Work out the finished part from the listing and answer in its coordinate system (mm). A direction names the side the tool comes from. Round coordinates to 2 decimals unless told otherwise and drop trailing zeros. Order: outer loops, then holes, each group sorted by start corner. A loop starts at its lowest first (then second) coordinate and runs counter-clockwise, first axis right, second up. Notation, with made-up numbers: (75.5, -13.5) - (80.5, -13.5) arc R35 ccw to (80.5, 25.5) - close; hole circle Ø6 at (31.25, 85). An arc over 180 degrees is marked (long way). Use one line per item in the form item = value. Start each with the question number.
Q1. Find the intervals of material crossed by line 1 (Z direction, x = 100, y = 1.55); line 2 (Z direction, x = 6, y = 2.05); line 3 (X direction, y = 0.8, z = -65), in increasing order. Write a range as [from, to].
Q2. Which of the six approach directions +Z, -Z, +X, -X, +Y, -Y give full straight-line access (tool end or side, diameter ignored) to faces 1 (the cylindrical face through (-92.85, 1.48, -71.89)), 2 (the flat face through (-134.558, 1.479, 0.347))?
Q3. For a pull along X with two mould halves and no side action, classify faces 3 (the flat face through (-2, 3, -3)), 4 (the flat face through (134.17, 1.48, 0.91)), 5 (the cylindrical face through (87.15, 1.48, -47.91)) as +X half, -X half, draft (parallel to the pull), parting line (faces both ways), or undercut.
Q4. The part is cut by section A-A on x = 0. Determine the outline of the cut face in (y, z), plus the area to 4 significant figures.
Q5. Given P1, Ø1.5, axis at x = -8, y = 1.5, coming from the -Z side; P2, Ø1.5, axis at y = 1.5, z = -21.5, coming from the -X side; P3, Ø0.9, axis at x = -126.5, y = 1.5, coming from the -Z side, each flat-ended and moving along its own axis, determine where each tip first touches the part or whether it passes through.
Q6. The part is cut by section C-C on x = 34. Determine the outline of the cut face in (y, z), plus the area to 3 significant figures.
Q7. The part is cut by section B-B on y = 1.3. State how many separate pieces and enclosed holes the cut face has, plus the area to 3 significant figures.
from build123d import *

# Parameters (mm, degrees)
EXTRUDE_1_DEPTH     = 3
SKETCH_2_R          = 1.75
CUT_EXTRUDE_1_DEPTH = 10
CUT_EXTRUDE_2_DEPTH = 3
SKETCH_4_R          = 9
CUT_EXTRUDE_3_DEPTH = 10
SKETCH_5_R          = 2.1
CUT_EXTRUDE_4_DEPTH = 4


with BuildPart() as part:
    # 草图1 → 凸台-拉伸1 (new body)
    with BuildSketch(Plane(origin=(0, 0, 0), x_dir=(1, 0, 0), z_dir=(0, 1, 0))):
        with BuildLine():
            Line((-148.235829522, 19.513411872), (-120.492131082, -20.771152042))
            ThreePointArc((-120.492131082, -20.771152042), (-116.908205257, -23.951300285), (-112.25630156, -25.099193643))
            Line((-112.25630156, -25.099193643), (112.25630156, -25.099193643))
            ThreePointArc((112.25630156, -25.099193643), (116.908205257, -23.951300285), (120.492131082, -20.771152042))
            Line((120.492131082, -20.771152042), (148.235829522, 19.513411872))
            ThreePointArc((148.235829522, 19.513411872), (149.548777283, 22.215378286), (150, 25.185370271))
            Line((150, 25.185370271), (150, 65))
            ThreePointArc((150, 65), (147.169490918, 72.124628896), (140.101052961, 75.092675968))
            Line((140.101052961, 75.092675968), (100.001859318, 75.092675968))
            ThreePointArc((100.001859318, 75.092675968), (92.860872953, 72.096900105), (90, 64.900806357))
            Line((90, 64.900806357), (90, 54.900806357))
            ThreePointArc((90, 54.900806357), (87.071067812, 47.829738545), (80, 44.900806357))
            Line((80, 44.900806357), (-80, 44.900806357))
            ThreePointArc((-80, 44.900806357), (-87.071067812, 47.829738545), (-90, 54.900806357))
            Line((-90, 54.900806357), (-90, 64.900806357))
            ThreePointArc((-90, 64.900806357), (-92.928932188, 71.971874169), (-100, 74.900806357))
            Line((-100, 74.900806357), (-140.099193643, 74.900806357))
            ThreePointArc((-140.099193643, 74.900806357), (-147.100120957, 72.000927314), (-150, 65))
            Line((-150, 65), (-150, 25.185370271))
            ThreePointArc((-150, 25.185370271), (-149.548777283, 22.215378286), (-148.235829522, 19.513411872))
        make_face()
    extrude(amount=EXTRUDE_1_DEPTH)

    # 草图2 → 切除-拉伸1 (cut)
    with BuildSketch(Plane(origin=(0, 3, 0), x_dir=(1, 0, 0), z_dir=(0, 1, 0))):
        with Locations(Location((100, 9.900806357, 0), (0, 0, 270))):
            Circle(SKETCH_2_R)
        with Locations(Location((100, -10.099193643, 0), (0, 0, 270))):
            Circle(SKETCH_2_R)
        with Locations(Location((-100, -10.099193643, 0), (0, 0, 90))):
            Circle(SKETCH_2_R)
        with Locations(Location((-100, 9.900806357, 0), (0, 0, 90))):
            Circle(SKETCH_2_R)
    extrude(amount=-CUT_EXTRUDE_1_DEPTH, mode=Mode.SUBTRACT)

    # 草图3 → 切除-拉伸2 (cut)
    with BuildSketch(Plane(origin=(0, 3, 0), x_dir=(1, 0, 0), z_dir=(0, 1, 0))):
        with BuildLine():
            Line((-10, 39.900806357), (10, 39.900806357))
            ThreePointArc((10, 39.900806357), (11.75, 38.150806357), (10, 36.400806357))
            Line((10, 36.400806357), (-10, 36.400806357))
            ThreePointArc((-10, 36.400806357), (-11.75, 38.150806357), (-10, 39.900806357))
        make_face()
    extrude(amount=-CUT_EXTRUDE_2_DEPTH, mode=Mode.SUBTRACT)

    # 草图4 → 切除-拉伸3 (cut)
    with BuildSketch(Plane(origin=(0, 3, 0), x_dir=(1, 0, 0), z_dir=(0, 1, 0))):
        with Locations(Location((0, 18.185077605, 0), (0, 0, 270))):
            Circle(SKETCH_4_R)
    extrude(amount=-CUT_EXTRUDE_3_DEPTH, mode=Mode.SUBTRACT)

    # 草图5 → 切除-拉伸4 (cut)
    with BuildSketch(Plane.XZ):
        with Locations(Location((-20.323459578, 2.138381974, 0), (0, 0, 270))):
            Circle(SKETCH_5_R)
        with Locations(Location((20.323459578, 2.138381974, 0), (0, 0, 270))):
            Circle(SKETCH_5_R)
        with Locations(Location((20.323459578, -38.508537183, 0), (0, 0, 270))):
            Circle(SKETCH_5_R)
        with Locations(Location((-20.323459578, -38.508537183, 0), (0, 0, 270))):
            Circle(SKETCH_5_R)
    extrude(amount=-CUT_EXTRUDE_4_DEPTH, mode=Mode.SUBTRACT)


solid = part.part
Found:
q1.line_1 = [-75.09, -11.65], [-8.15, 8.35], [11.85, 25.1]
q1.line_2 = [-44.9, -39.9], [-36.4, -24.89], [-11.48, 25.1]
q1.line_3 = [-150, -90], [90, 150]
q2.face_1 = -Z, +Y, -Y
q2.face_2 = +Z, -X, +Y, -Y
q3.face_3 = draft
q3.face_4 = +X half
q3.face_5 = undercut
q4.outline = (0, -44.9) - (3, -44.9) - (3, -39.9) - (0, -39.9) - close; (0, -36.4) - (3, -36.4) - (3, -27.19) - (0, -27.19) - close; (0, -9.19) - (3, -9.19) - (3, 25.1) - (0, 25.1) - close
q4.area = 145.5 mm²
q5.P1 = -44.9
q5.P2 = -149.56
q5.P3 = -74.9
q6.outline = (0, -44.9) - (3, -44.9) - (3, 25.1) - (0, 25.1) - close
q6.area = 210 mm²
q7.separate_pieces = 1
q7.enclosed_holes = 10
q7.area = 22,600 mm²
